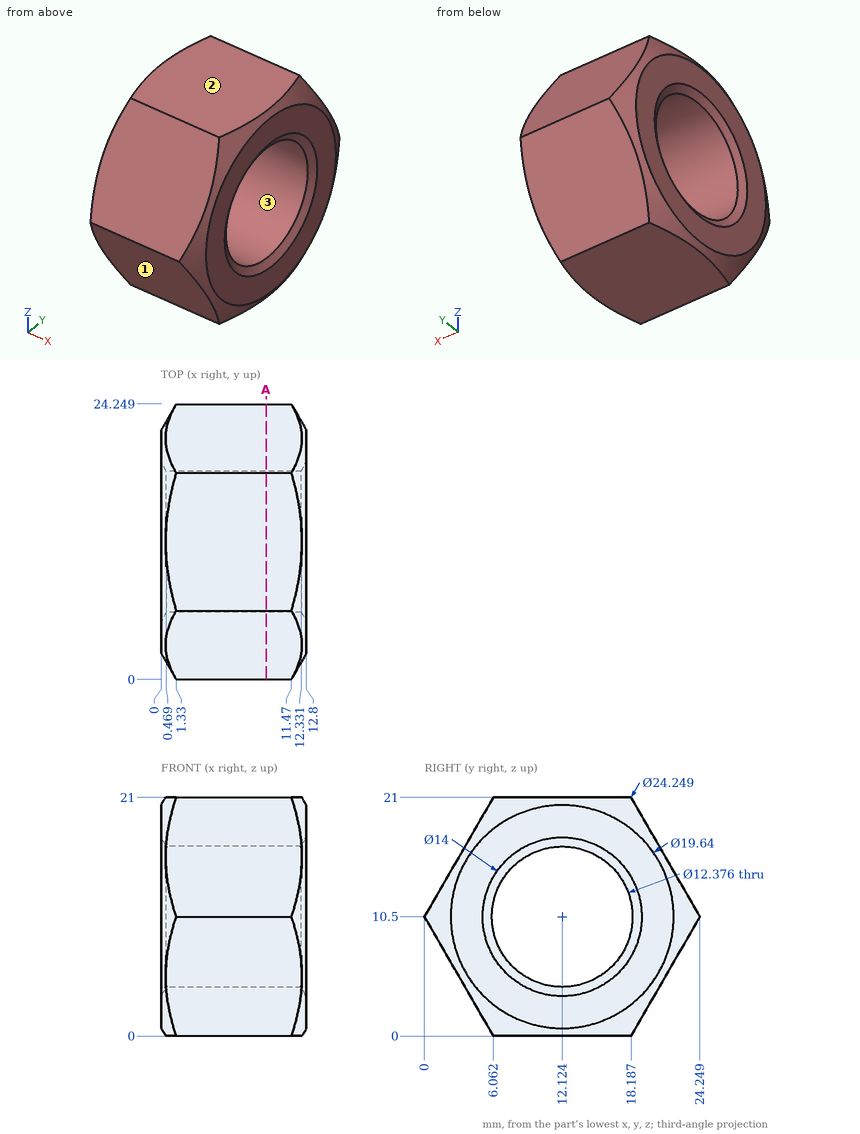
Study the drawing (mm; zero at the part's minimum x, y, z) and answer. Give positions to 0.01 mm unless a question says otherwise; leave off trailing zeros. Write each loop counter-clockwise with the first axis right and the second up, starting at its lowest first coordinate (ties: lowest second). Pieces come first, ordered by that corner, then holes.
Item 1: Section A-A, the plane x = 9.25 is taken. Write down the section's boundary in (y, z) (1 decimal), plus the area to 3 significant figures.
Item 2: Determine the mould class of the marked faces 1, 2 and 3 for opening direction Y: released by +Y, released by -Y, zero draft, split by the parting line, or undercut.
Item 3: Flat-ended cylindrical pins translate along their axes: P1, Ø11, axis at y = 12.12, z = 10.5, coming from the +X side; P2, Ø2, axis at x = 1.5, z = 4, coming from the +Y side. Find the tip coordinate at first contact, or state that the pin passes through.
Item 4: Find the intervals of material crossed by line 1 along Z through (x, y) = (9.25, 7); line 2 along Y through (x, z) = (2, 12.75); line 3 along Y through (x, z) = (5.25, 11.75) (1 decimal), in increasing order.
Completed:
1. outline: (0, 10.5) - (6.1, 0) - (18.2, 0) - (24.2, 10.5) - (18.2, 21) - (6.1, 21) - close; hole circle Ø12.4 at (12.1, 10.5)
1. area: 262 mm2
2. face 1: released by -Y
2. face 2: zero draft
2. face 3: undercut
3. P1: passes through
3. P2: stops at y = 21.07
4. line 1: z = 0 to 7.03, 13.97 to 21
4. line 2: y = 1.3 to 6.36, 17.89 to 22.95
4. line 3: y = 0.7 to 6.1, 18.2 to 23.5
